For this review, use the dimensioned drawing (mm, ordinates from the lowest corner) and the shaded views. Give positions to 0.01 mm unless a question says otherwise; leave off trailing zeros. Loops run counter-clockwise (first coordinate to the right, second up) from the corner with the lowest first, then second, coordinate; pieces in that order, holes last. Notation, with made-up numbers: (79.25, 61) -> (97.25, 61) arc R32 cw to (97.25, 93) -> close; hole circle Ø6 at (-30.75, 5.25). An arc over 180 degrees is marked (long way). Write each question's results on one line, items separated by ' | '. Start each with the question number.
Q1. We need section A-A (x = 173). Write out the cut boundary in (y, z), plus the area to 3 significant figures.
Q2. We need section B-B (y = 99). Write out the cut boundary in (x, z).
Q3. Insertion check: pin 1 Ø2 at (y, z) = (31, 13) entering from -X; pin 2 Ø8 at (x, z) = (165, 4) entering from -Y; pin 3 Ø1 at (x, z) = (140.5, 15) entering from -Y; pin 4 Ø5 at (x, z) = (39, 3.5) entering from +Y. Each pin has a flat end and moves straight along its axis. Give the tip position at first contact, or say it passes through.
Q4. Wall thickness on L1, parallel to Z at x = 43, y = 13.5; L2, parallel to Z at x = 74, y = 17.5; L3, parallel to Y at x = 27, z = 10.25 (1 decimal): over which ranges is each line inside the solid? List them lowest first. Write a range as [from, to].
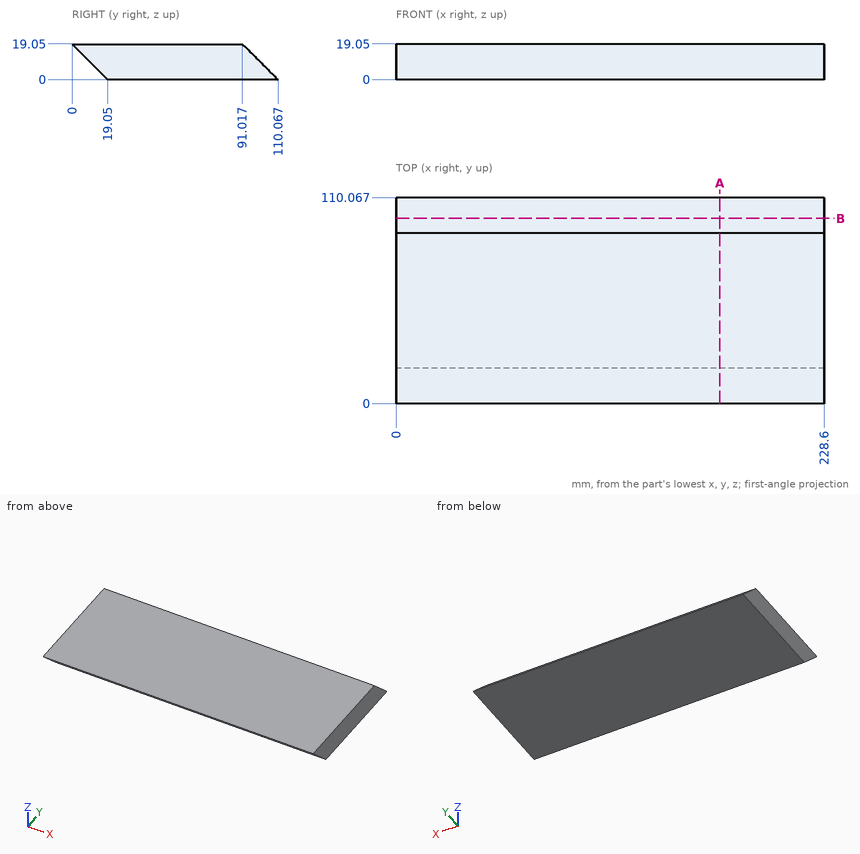
Output:
1) outline: (0, 19.05) -> (19.05, 0) -> (110.07, 0) -> (91.02, 19.05) -> close | area: 1,730 mm2
2) outline: (0, 0) -> (228.6, 0) -> (228.6, 11.07) -> (0, 11.07) -> close
3) pin 1: x = 0 | pin 2: y = 11.05 | pin 3: y = 3.55 | pin 4: y = 109.07
4) L1: [5.55, 19.05] | L2: [1.55, 19.05] | L3: [8.8, 99.8]
